from build123d import *

# Parameters (mm, degrees)
SKETCH_1_W          = 52
SKETCH_1_H          = 46
EXTRUDE_1_DEPTH     = 12
SKETCH_2_W          = 52
SKETCH_2_H          = 23
EXTRUDE_2_DEPTH     = 12
SKETCH_3_R          = 2.5
CUT_EXTRUDE_1_DEPTH = 74.457470689
SKETCH_4_W          = 24
SKETCH_4_H          = 1
CUT_EXTRUDE_2_DEPTH = 71.455659815


with BuildPart() as part:
    # 草图1 → 凸台-拉伸1 (new body)
    with BuildSketch(Plane(origin=(0, 0, 0), x_dir=(1, 0, 0), z_dir=(0, 1, 0))):
        with Locations((26, 23)):
            Rectangle(SKETCH_1_W, SKETCH_1_H)
    extrude(amount=EXTRUDE_1_DEPTH)

    # 草图2 → 凸台-拉伸2 (add)
    with BuildSketch(Plane.XZ):
        with Locations((26, -23)):
            Rectangle(SKETCH_2_W, SKETCH_2_H)
    extrude(amount=EXTRUDE_2_DEPTH)

    # 草图3 → 切除-拉伸1 (cut, through all)
    with BuildSketch(Plane(origin=(0, 12, 0), x_dir=(1, 0, 0), z_dir=(0, 1, 0))):
        with Locations(Location((8, 39, 0), (0, 0, 270))):
            Circle(SKETCH_3_R)
        with Locations(Location((8, 7, 0), (0, 0, 90))):
            Circle(SKETCH_3_R)
        with Locations(Location((44, 7, 0), (0, 0, 270))):
            Circle(SKETCH_3_R)
        with Locations(Location((44, 39, 0), (0, 0, 90))):
            Circle(SKETCH_3_R)
    extrude(amount=-CUT_EXTRUDE_1_DEPTH, mode=Mode.SUBTRACT)

    # 草图4 → 切除-拉伸2 (cut, through all)
    with BuildSketch(Plane.ZY):
        with Locations((-23, 11.5)):
            Rectangle(SKETCH_4_W, SKETCH_4_H)
    extrude(amount=-CUT_EXTRUDE_2_DEPTH, mode=Mode.SUBTRACT)


solid = part.part
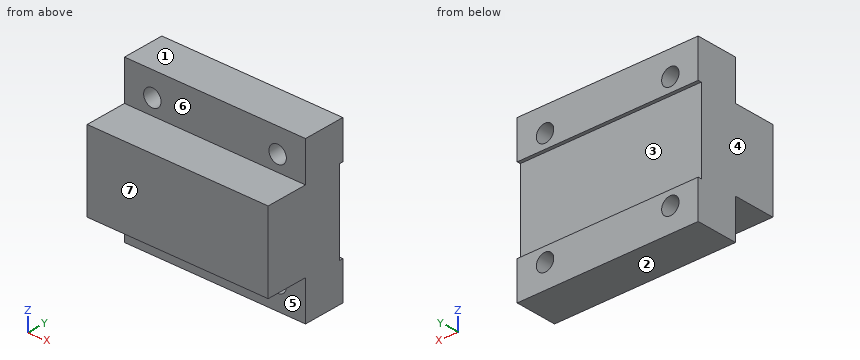
The model under review builds one solid part; all positions refer to its coordinate system, in mm. Face numbers are marked on the shaded views. A direction names the side the tool comes from. Give positions to 0.01 mm unless a question says otherwise; leave off trailing zeros. Loops run counter-clockwise (first coordinate to the right, second up) from the corner with the lowest first, then second, coordinate; pieces in that order, holes last. Notation, with made-up numbers: (64, 68) -> (91, 68) arc R14 cw to (91, 94) -> close; hole circle Ø4 at (-18.75, 7). An arc over 180 degrees is marked (long way). Answer as a JSON object with one key per item and string values. Group by question number.
Q1. Take a section at B-B (x = 8). Write out the cut boundary in (y, z).
Q2. Tool access review of the marked faces 5, 6 and 7: name each direction out of +Z, -Z, +X, -X, +Y, -Y from which nothing blocks a thin tool from reaching the whole face with its end or side.
Q3. Take a section at D-D (z = -3.5). Write out the cut boundary in (x, y), plus the area to 3 significant figures.
Q4. Wall thickness on line 1 along X through (y, z) = (3, -39); line 2 along Y through (x, z) = (19, -12); line 3 along Y through (x, z) = (41.5, -10): over which ranges is each line inside the solid? List them lowest first.
Q5. Draft analysis for pull direction Z (two halves, no side actions). For the marked faces 1, 2, 3 and 4, state which applies: pulls with the +Z half, pulls with the -Z half, needs draft (parallel to the pull), parting line crosses it, or undercut.
Q6. Take a section at A-A (z = -39). Write out the cut boundary in (x, y).
Q7. Insertion check: pin 1 (2 mm diameter, centred on x = 38.5, z = -6, fed in from -Y); pin 2 (6 mm diameter, centred on x = 38.5, y = -3.5, fed in from -Z); pin 3 (1 mm diameter, centred on x = 7.5, z = -5.5, fed in from +Y); pin 4 (7 mm diameter, centred on x = 29.5, z = -21, fed in from +Y). Each pin has a flat end and moves straight along its axis. Give the tip position at first contact, or say it passes through.
Q8. Take a section at C-C (y = -1.5). Write out the cut boundary in (x, z), plus the area to 3 significant figures.
Answer below:
{
 "1": {"outline": "(-12, -34.5) -> (0, -34.5) -> (0, -36.5) -> (12, -36.5) -> (12, -35) -> (11, -35) -> (11, -11) -> (12, -11) -> (12, -9.5) -> (0, -9.5) -> (0, -11.5) -> (-12, -11.5) -> close; (0, -46) -> (12, -46) -> (12, -41.5) -> (0, -41.5) -> close; (0, -4.5) -> (12, -4.5) -> (12, 0) -> (0, 0) -> close"},
 "2": {"face 5": "-Z, +X, -X, -Y", "face 6": "+Z, +X, -X, -Y", "face 7": "+Z, -Z, +X, -X, -Y"},
 "3": {"outline": "(0, 0) -> (52, 0) -> (52, 12) -> (0, 12) -> close", "area": "624 mm2"},
 "4": {"line 1": "x = 0 to 5.5, 10.5 to 41.5, 46.5 to 52", "line 2": "y = -12 to 11", "line 3": "y = 0 to 12"},
 "5": {"face 1": "pulls with the +Z half", "face 2": "pulls with the -Z half", "face 3": "undercut", "face 4": "needs draft"},
 "6": {"outline": "(0, 0) -> (5.5, 0) -> (5.5, 12) -> (0, 12) -> close; (10.5, 0) -> (41.5, 0) -> (41.5, 12) -> (10.5, 12) -> close; (46.5, 0) -> (52, 0) -> (52, 12) -> (46.5, 12) -> close"},
 "7": {"pin 1": "stops at y = 0", "pin 2": "stops at z = -34.5", "pin 3": "passes through", "pin 4": "stops at y = 11"},
 "8": {"outline": "(0, -34.5) -> (52, -34.5) -> (52, -11.5) -> (0, -11.5) -> close", "area": "1,200 mm2"}
}
